Geometry: see drawing. Coordinates: mm, zero at the bounding-box minimum. Coordinates: 2 decimals unless noted, no trailing zeros. Loops run counter-clockwise (first coordinate to the right, second up) from the corner with the lowest first, then second, coordinate; pieces in that order, holes last. Notation, with made-up numbers: (15.25, 24) - (61.25, 24) arc R9 cw to (61.25, 28) - close; hole circle Ø6 at (-29, 78). An arc over 180 degrees is marked (long way). Answer in a Markdown table with one row per item.
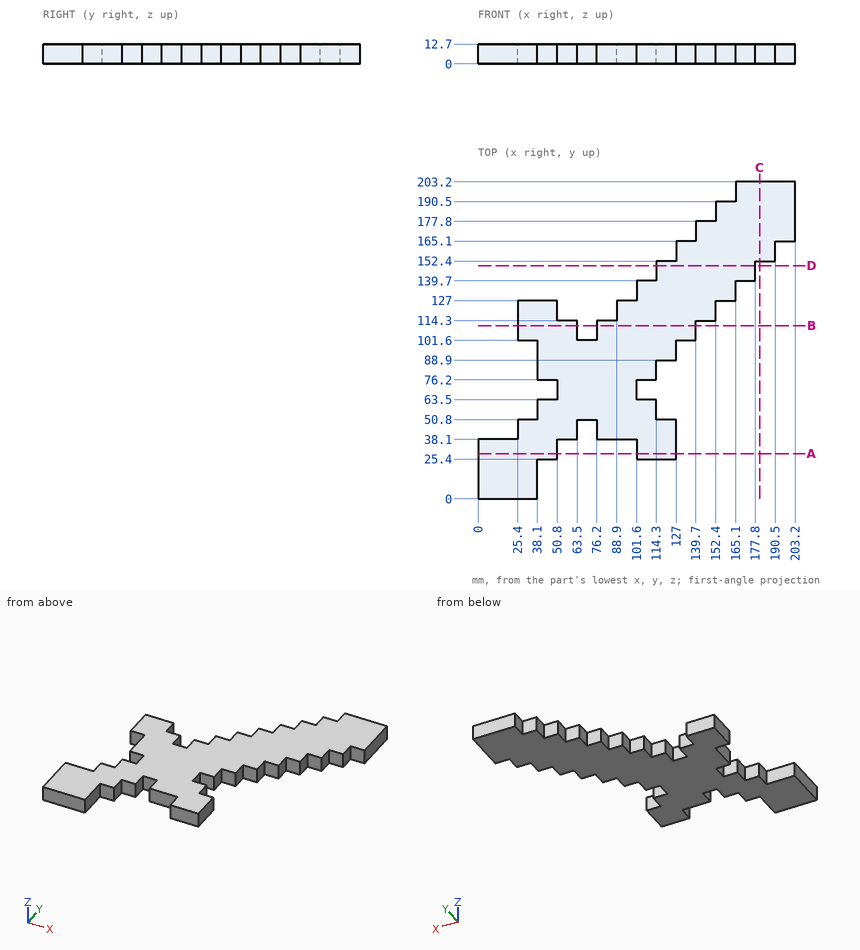
(1) Cut plane B-B on y = 111. Output: boundary loops of the cut face in (x, z).
Verdict:
| item | result |
|---|---|
| outline | (25.4, 0) - (63.5, 0) - (63.5, 12.7) - (25.4, 12.7) - close; (76.2, 0) - (139.7, 0) - (139.7, 12.7) - (76.2, 12.7) - close |
(2) Cut plane A-A on y = 29. Output: boundary loops of the cut face in (x, z), then the cut area to 3 significant figures.
Verdict:
| item | result |
|---|---|
| outline | (0, 0) - (50.8, 0) - (50.8, 12.7) - (0, 12.7) - close; (101.6, 0) - (127, 0) - (127, 12.7) - (101.6, 12.7) - close |
| area | 968 mm² |
(3) First-contact query: pin 1 Ø4 at (x, z) = (88.5, 8.5) entering from -Y; pin 2 Ø5 at (x, z) = (51, 10.5) entering from +Y; pin 3 Ø4 at (x, z) = (171.5, 3.5) entering from -Y. Flat tips, straight axial feed; report the tip coordinate or a pass-through.
Verdict:
| item | result |
|---|---|
| pin 1 | stops at y = 38.1 |
| pin 2 | stops at y = 127 |
| pin 3 | stops at y = 139.7 |
(4) Ray query, probe 1 along Y at (x, z) = (119.5, 6.5); probe 2 along Y at (x, z) = (109, 0.5). Return the intervals inside material, ascending.
Verdict:
| item | result |
|---|---|
| probe 1 | y = 25.4 to 50.8, 88.9 to 152.4 |
| probe 2 | y = 25.4 to 63.5, 76.2 to 139.7 |
(5) Cut plane C-C on x = 180.5. Output: boundary loops of the cut face in (y, z).
Verdict:
| item | result |
|---|---|
| outline | (152.4, 0) - (203.2, 0) - (203.2, 12.7) - (152.4, 12.7) - close |
(6) Cut plane D-D on y = 149.5. Output: boundary loops of the cut face in (x, z), then the cut area to 3 significant figures.
Verdict:
| item | result |
|---|---|
| outline | (114.3, 0) - (177.8, 0) - (177.8, 12.7) - (114.3, 12.7) - close |
| area | 806 mm² |
